Model file for the job. Use its own axes, mm. A direction names the side the tool comes from. Give positions to 0.01 mm unless a question says otherwise; leave off trailing zeros. Write each loop counter-clockwise with the first axis right and the second up, starting at its lowest first coordinate (ties: lowest second). Pieces come first, ordered by that corner, then holes. Notation, with made-up numbers: (-31, 71) - (12, 71) arc R30 cw to (12, 104) - close; hole circle Ø3 at (-8.5, 21). An arc over 180 degrees is marked (long way). One line per item, written item: value. Start each with the question number.
(1) Cut at D-D, the plane x = 13. List the corners of the cut face in (y, z).
(2) Cut at A-A, the plane z = 3.4. List the corners of the cut face in (x, y).
(3) Cut at B-B, the plane x = 22.5. List the corners of the cut face in (y, z).
(4) 3-axis set-ups, long thin cutter, end or side, ignore diameter. For faces 4 (the face through (15, 25, 2.5)), 5 (the face through (22, 0, 2)): which of +Z, -Z, +X, -X, +Y, -Y reach the whole face in a straight line?
(5) Probe L1, parallel to Y at x = 22.5, z = 4.55; L2, parallel to Z at x = 30, y = 27. List the from-to ranges inside material, lowest first.
(6) Mould opens along X. For faces 1 (the face through (45, 22, 2)), 2 (the face through (16.32, 12.8, 3.77)), 3 (the face through (23, 45, 2)) say: pulls with the +X half, pulls with the -X half, needs draft (parallel to the pull), parting line crosses it, or undercut.
Autodesk Fusion 360 part; units mm, degrees
sketch "Sketch1" plane through (0, 0, 0) normal (0, 0, 1) x (1, 0, 0)
  line L0 (0, 0) -> (45, 0)
  line L1 (45, 0) -> (45, 45)
  line L2 (45, 45) -> (0, 45)
  line L3 (0, 45) -> (0, 0)
  dimension "d1" = 45
  dimension "d2" = 45
extrude "Extrude1" add sketch "Sketch1" along normal blind 5
sketch "Sketch2" plane through (0, 0, 5) normal (0, 0, 1) x (-1, 0, 0)
  line L0 (0, -45) -> (0, 0)
  line L1 (0, 0) -> (-45, 0)
  line L2 (-45, 0) -> (-45, -50)
  line L3 (-45, -45) -> (0, -45)
  line L4 (0, -45) -> (-45, -45)
  line L5 (-45, -45) -> (-45, -50)
  line L6 (-45, -50) -> (0, -50)
  line L7 (0, -50) -> (0, -45)
  line L8 (0, 0) -> (-45, 0)
  line L9 (-45, 0) -> (-45, 5)
  line L10 (-45, 5) -> (0, 5)
  line L11 (0, 5) -> (0, 0)
  line L12 (0, -50) -> (-45, 5)
  line L13 (-45, -50) -> (0, 5)
  circle A0 centre (-22.5, -22.5) radius 7.5
  circle A1 centre (-22.5, -22.5) radius 11.5
  dimension "d5" = 45
  dimension "d6" = 5
  dimension "d7" = 45
  dimension "d8" = 5
  dimension "d13" = 15
  dimension "d14" = 23
extrude "Extrude3" cut sketch "Sketch2" against normal blind 2.5 contours L12 L13 A0 A1 | L12 L13 A0 A1 | L12 L13 A0 A1 | L12 L13 A0 A1
Answers follow:
1. outline: (0, 0) - (45, 0) - (45, 5) - (28.98, 5) - (28.98, 2.5) - (16.02, 2.5) - (16.02, 5) - (0, 5) - close
2. outline: (0, 0) - (45, 0) - (45, 45) - (0, 45) - close; circle Ø15 at (22.5, 22.5); hole circle Ø23 at (22.5, 22.5)
3. outline: (0, 0) - (45, 0) - (45, 5) - (34, 5) - (34, 2.5) - (30, 2.5) - (30, 5) - (15, 5) - (15, 2.5) - (11, 2.5) - (11, 5) - (0, 5) - close
4. face 4: +Z
4. face 5: +Z, -Z, +X, -X, -Y
5. L1: y = 0 to 11, 15 to 30, 34 to 45
5. L2: z = 0 to 2.5
6. face 1: pulls with the +X half
6. face 2: undercut
6. face 3: needs draft
